Here's how the part is built. I have some questions about the finished solid (model axes, mm). A direction names the side the tool comes from. Round coordinates to 2 decimals unless told otherwise and drop trailing zeros. Write each loop counter-clockwise with the first axis right and the second up, starting at its lowest first coordinate (ties: lowest second). Pieces come first, ordered by that corner, then holes. Notation, with made-up numbers: (35, -12) - (63, -12) arc R24 ccw to (63, 10) - close; hole circle Ø9 at (-31, 59.5). An arc over 180 degrees is marked (long way). Use one line per item in the form item = value. Start each with the question number.
1. I want a section at A-A, the plane y = -1.75. List the corners of the cut face in (x, z) for me.
2. I want a section at B-B, the plane z = -9. List the corners of the cut face in (x, y) for me, plus the area to 3 significant figures.
3. We'd pull the mould along X, two halves only. Please class faces 1 (the flat face through (-11.769, 4.93, -11.005)), 2 (the flat face through (28, 20, -11)): +X half, -X half, draft (parallel to the pull), parting line (faces both ways), or undercut.
4. Will these pins go through, and if not, where does the flat tip stop? pin 1 (8.5 mm diameter, centred on x = -11.78, z = -15.92, fed in from -Y); pin 2 (12 mm diameter, centred on x = 2.5, y = 9.5, fed in from +Z); pin 3 (4 mm diameter, centred on x = -11, z = -25.5, fed in from +Y).
5. If I drill on line 1 along X through (y, z) = (6, -21); line 2 along Y through (x, z) = (-6, -26.5); line 3 along Z through (x, y) = (-11, 4.25), over which ranges is the centre line in solid material (lowest first)?
6. Which directions (+Z, -Z, +X, -X, +Y, -Y) give clear straight access to the entire face, cutting with the end or side of a thin tool? Please do faces 3 (the cylindrical face through (33.994, 5.21, -14.395)), 4 (the cylindrical face through (-9.45, 7.92, -32.02)), 5 (the flat face through (28, -10, -11)).
```python
from build123d import *

# Parameters (mm, degrees)
EXTRUDE_THIN1_DEPTH = 10
SKETCH3_R           = 6.920707693
BOSS_EXTRUDE1_DEPTH = 10
BOSS_EXTRUDE3_START = -30
SKETCH6_R           = 6.920707693
BOSS_EXTRUDE3_DEPTH = 30
FILLET5_R           = 3
CUT_EXTRUDE2_DEPTH  = 4.2291
SKETCH8_R           = 1
CUT_EXTRUDE3_DEPTH  = 10


# Read off the part's stored shape, not the designer's step: Extrude-Thin1
with BuildPart() as part:
    # Extrude-Thin1 outline → Extrude-Thin1 (new body)
    with BuildSketch(Plane(origin=(0, 0, 0), x_dir=(1, 0, 0), z_dir=(0, 1, 0))):
        with BuildLine():
            Line((22.787644573, 16.321054497), (32.786727129, 16.185599595))
            add(Edge.make_bspline(
                [(32.786727129, 16.185599595), (32.811960434, 18.048285218), (32.641015725, 19.879615359), (31.92970267, 23.402358796), (31.389692113, 25.092847565), (29.996264529, 28.265553908), (29.143647795, 29.747564833), (27.19528421, 32.464868479), (26.100039873, 33.700572008), (23.728981302, 35.912471104), (22.453221171, 36.889166895), (19.767583781, 38.580346198), (18.357513706, 39.295168947), (15.436486932, 40.456738309), (13.925220488, 40.90365338), (10.829703301, 41.512793064), (9.245032555, 41.674991243), (6.03621689, 41.684984578), (4.411608755, 41.532400863), (1.175780595, 40.875380655), (-0.435544855, 40.370107305), (-3.562076247, 38.980716277), (-5.076448982, 38.095842257), (-7.905525663, 35.957656136), (-9.218857585, 34.704759204), (-11.55775534, 31.887270708), (-12.582900642, 30.324085176), (-14.305177479, 26.958999197), (-15.003087647, 25.157977385), (-16.072049137, 21.36655254), (-16.443959592, 19.376041131), (-16.874579144, 15.219557311), (-16.93365201, 13.053120971), (-16.839375878, 10.793799857)],
                knots=[0, 0, 0, 0, 0.0625, 0.0625, 0.125, 0.125, 0.1875, 0.1875, 0.25, 0.25, 0.3125, 0.3125, 0.375, 0.375, 0.4375, 0.4375, 0.5, 0.5, 0.5625, 0.5625, 0.625, 0.625, 0.6875, 0.6875, 0.75, 0.75, 0.8125, 0.8125, 0.875, 0.875, 0.9375, 0.9375, 1, 1, 1, 1], degree=3))
            Line((-16.839375878, 10.793799857), (-6.848070504, 11.210713427))
            add(Edge.make_bspline(
                [(22.787644573, 16.321054497), (23.040705887, 35.001670137), (-8.061946573, 40.30117097), (-6.848070504, 11.210713427)],
                knots=[0, 0, 0, 0, 1, 1, 1, 1], degree=3))
        make_face()
    extrude(amount=EXTRUDE_THIN1_DEPTH)

    # Sketch3 → Boss-Extrude1 (add)
    with BuildSketch(Plane.XZ):
        with Locations(Location((27.722370723, -11.46876918, 0), (0, 0, 317.034865558))):
            Circle(SKETCH3_R)
    extrude(amount=BOSS_EXTRUDE1_DEPTH)

    # Sketch6 → Boss-Extrude3 (add)
    with BuildSketch(Plane.XZ.offset(10).offset(BOSS_EXTRUDE3_START)):
        with Locations(Location((27.722370723, -11.46876918, 0), (0, 0, 270))):
            Circle(SKETCH6_R)
    extrude(amount=BOSS_EXTRUDE3_DEPTH)

    # Fillet5
    fillet5_edges = [part.edges().sort_by_distance(p)[0] for p in [
        (-6.848070504, 5, -11.210713427),
        (-16.839375878, 5, -10.793799857),
    ]]
    fillet(fillet5_edges, radius=FILLET5_R)

    # Sketch7 → Cut-Extrude2 (cut)
    with BuildSketch(Plane(origin=(0, 10, -10), x_dir=(1, 0, 0), z_dir=(0, -1, 0))):
        with BuildLine():
            Line((-8.649516125, -7.733026517), (-7.738756929, -19.897223008))
            ThreePointArc((-7.738756929, -19.897223008), (-9.492313797, -22.025587149), (-11.58447009, -20.228985455))
            Line((-11.58447009, -20.228985455), (-14.488068719, -8.331888199))
            ThreePointArc((-14.488068719, -8.331888199), (-12.154290458, -2.324192527), (-8.649516125, -7.733026517))
        make_face()
    extrude(amount=CUT_EXTRUDE2_DEPTH, mode=Mode.SUBTRACT)

    # Sketch8 → Cut-Extrude3 (cut)
    with BuildSketch(Plane(origin=(0, 5.7709, 0), x_dir=(1, 0, 0), z_dir=(0, 1, 0))):
        with Locations(Location((-11.784975147, 15.924801705, 0), (0, 0, 270))):
            Circle(SKETCH8_R)
    extrude(amount=-CUT_EXTRUDE3_DEPTH, mode=Mode.SUBTRACT)


solid = part.part
```
Model answer:
q1.outline = circle Ø13.84 at (27.72, -11.47)
q2.outline = (21.26, -10) - (34.19, -10) - (34.19, 20) - (21.26, 20) - close
q2.area = 388 mm2
q3.face_1 = undercut
q3.face_2 = draft
q4.pin_1 = 0
q4.pin_2 = -25.84
q4.pin_3 = 10
q5.line_1 = -16.09 to -13.84, -8.4 to -5.78, 22.15 to 32.41
q5.line_2 = 0 to 10
q5.line_3 = -32.53 to -16.54, -15.31 to -11.04
q6.face_3 = none
q6.face_4 = +Y
q6.face_5 = +Z, -Z, +X, -X, -Y
